Geometry: final body of the model. Coordinates: model frame, mm. A direction names the side the tool comes from. Give positions to 0.01 mm unless a question says otherwise; leave off trailing zeros. Order: outer loops, then holes, each group sorted by start corner. A loop starts at its lowest first (then second) coordinate and runs counter-clockwise, first axis right, second up. Notation, with made-up numbers: (9, 34) - (48, 34) arc R29 cw to (48, 60) - close; hole circle Ø5 at (60, 70). An arc over 180 degrees is marked (long way). Use one line per item in the form item = value.
from build123d import *

# Parameters (mm, degrees)
F0_W     = 177.8
F0_H     = 165.1
F1_DEPTH = 6.35
F2_W     = 190.5
F2_H     = 177.8
F2_W_2   = 177.8
F2_H_2   = 165.1
F3_DEPTH = 50.8


with BuildPart() as f1:
    # F0 (on Top) → F1 (new body)
    with BuildSketch(Plane.XY):
        Rectangle(F0_W, F0_H)
    extrude(amount=F1_DEPTH)

    # F2 (on Top) → F3 (join)
    with BuildSketch(Plane.XY):
        Rectangle(F2_W, F2_H)
        Rectangle(F2_W_2, F2_H_2, mode=Mode.SUBTRACT)
    extrude(amount=F3_DEPTH)


solid = f1.part
(1) Ray query, line 1 along Y through (x, z) = (30.5, 8.5); line 2 along X through (y, z) = (-55, 12); line 3 along Z through (x, y) = (59, 32.5). Return the intervals inside material, ascending.
Computed values:
line_1 = -88.9 to -82.55, 82.55 to 88.9
line_2 = -95.25 to -88.9, 88.9 to 95.25
line_3 = 0 to 6.35
(2) Cut plane B-B on y = -15.5. Output: boundary loops of the cut face in (x, z).
Computed values:
outline = (-95.25, 0) - (95.25, 0) - (95.25, 50.8) - (88.9, 50.8) - (88.9, 6.35) - (-88.9, 6.35) - (-88.9, 50.8) - (-95.25, 50.8) - close
(3) Reachability of faces 1 (the face through (-8, -85, 50.8)), 2 (the face through (-88.9, -1, 28)) from +Z, -Z, +X, -X, +Y, -Y: full face, straight path, thin tool, end or side. Return the list, or none.
Computed values:
face_1 = +Z, +X, -X, +Y, -Y
face_2 = +Z
(4) Cut plane A-A on z = 22.5. Output: boundary loops of the cut face in (x, y).
Computed values:
outline = (-95.25, -88.9) - (95.25, -88.9) - (95.25, 88.9) - (-95.25, 88.9) - close; hole (-88.9, -82.55) - (88.9, -82.55) - (88.9, 82.55) - (-88.9, 82.55) - close
(5) Cut plane C-C on x = -29. Output: boundary loops of the cut face in (y, z).
Computed values:
outline = (-88.9, 0) - (88.9, 0) - (88.9, 50.8) - (82.55, 50.8) - (82.55, 6.35) - (-82.55, 6.35) - (-82.55, 50.8) - (-88.9, 50.8) - close
(6) Contact query for a flat-ended pin moving along its axis: pin 1 Ø4 at (x, y) = (-34, 27.5) entering from +Z. Output: stop coordinate, or through.
Computed values:
pin_1 = 6.35
(7) Pull-direction query (Y, two-part tool) for faces 3 (the face through (-1, 88.9, 25)), 4 (the face through (95.25, -1, 25)), 5 (the face through (-1, -82.55, 28)), 6 (the face through (-1, -88.9, 25)); classes: released by +Y, released by -Y, zero draft, split by the parting line, or undercut.
Computed values:
face_3 = released by +Y
face_4 = zero draft
face_5 = undercut
face_6 = released by -Y
